Input: part model. Units: mm. Frame: model coordinates. A direction names the side the tool comes from. Coordinates: 2 decimals unless noted, no trailing zeros. Order: outer loops, then holes, each group sorted by start corner. A loop starts at its lowest first (then second) coordinate and runs counter-clockwise, first axis right, second up.
from build123d import *

# Parameters (mm, degrees)
SKETCH1_W           = 70
SKETCH1_H           = 30
BOSS_EXTRUDE1_DEPTH = 5
SKETCH2_W           = 70
SKETCH2_H           = 2
BOSS_EXTRUDE2_DEPTH = 50
SKETCH3_W           = 2
SKETCH3_H           = 26
BOSS_EXTRUDE3_DEPTH = 50
SKETCH4_W           = 42
SKETCH4_H           = 13
SKETCH4_W_2         = 40
SKETCH4_H_2         = 11
BOSS_EXTRUDE4_DEPTH = 40
SKETCH6_W           = 40
SKETCH6_H           = 40
CUT_EXTRUDE1_DEPTH  = 2
SKETCH7_W           = 15
SKETCH7_H           = 18
CUT_EXTRUDE2_DEPTH  = 5
SKETCH8_W           = 10
SKETCH8_H           = 10
CUT_EXTRUDE3_DEPTH  = 5


with BuildPart() as part:
    # Sketch1 → Boss-Extrude1 (new body)
    with BuildSketch(Plane(origin=(0, 0, 0), x_dir=(1, 0, 0), z_dir=(0, 1, 0))):
        Rectangle(SKETCH1_W, SKETCH1_H)
    extrude(amount=BOSS_EXTRUDE1_DEPTH)

    # Sketch2 → Boss-Extrude2 (add)
    with BuildSketch(Plane(origin=(0, 5, 0), x_dir=(1, 0, 0), z_dir=(0, 1, 0))):
        with Locations((0, -14)):
            Rectangle(SKETCH2_W, SKETCH2_H)
        with Locations((0, 14)):
            Rectangle(SKETCH2_W, SKETCH2_H)
    extrude(amount=BOSS_EXTRUDE2_DEPTH)

    # Sketch3 → Boss-Extrude3 (add)
    with BuildSketch(Plane(origin=(0, 5, 0), x_dir=(1, 0, 0), z_dir=(0, 1, 0))):
        with Locations((-34, 0)):
            Rectangle(SKETCH3_W, SKETCH3_H)
        with Locations((34, 0)):
            Rectangle(SKETCH3_W, SKETCH3_H)
    extrude(amount=BOSS_EXTRUDE3_DEPTH)

    # Sketch4 → Boss-Extrude4 (add)
    with BuildSketch(Plane(origin=(0, 5, 0), x_dir=(1, 0, 0), z_dir=(0, 1, 0))):
        Rectangle(SKETCH4_W, SKETCH4_H)
        Rectangle(SKETCH4_W_2, SKETCH4_H_2, mode=Mode.SUBTRACT)
    extrude(amount=BOSS_EXTRUDE4_DEPTH)

    # Sketch6 → Cut-Extrude1 (cut)
    with BuildSketch(Plane.XY.offset(6.5)):
        with Locations((0, 25)):
            Rectangle(SKETCH6_W, SKETCH6_H)
    extrude(amount=-CUT_EXTRUDE1_DEPTH, mode=Mode.SUBTRACT)

    # Sketch7 → Cut-Extrude2 (cut)
    with BuildSketch(Plane.XY.offset(15)):
        with Locations((-7.5, 36.5)):
            Rectangle(SKETCH7_W, SKETCH7_H)
        with Locations((7.5, 36.5)):
            Rectangle(SKETCH7_W, SKETCH7_H)
        with Locations((7.5, 18.5)):
            Rectangle(SKETCH7_W, SKETCH7_H)
        with Locations((-7.5, 18.5)):
            Rectangle(SKETCH7_W, SKETCH7_H)
    extrude(amount=-CUT_EXTRUDE2_DEPTH, mode=Mode.SUBTRACT)

    # Sketch8 → Cut-Extrude3 (cut)
    with BuildSketch(Plane.XZ):
        Rectangle(SKETCH8_W, SKETCH8_H)
    extrude(amount=-CUT_EXTRUDE3_DEPTH, mode=Mode.SUBTRACT)


solid = part.part
Item 1: Access query for faces 4 (the face through (0, 30, -13)), 5 (the face through (5, 2, 0)), 6 (the face through (15, 27, 14)). Directions: +Z, -Z, +X, -X, +Y, -Y. A direction counts if a zero-diameter tool reaches every point of the face in a straight line with its end or side. Return the directions, or none.
Response values:
face 4: +Y
face 5: +Y, -Y
face 6: +Z
Item 2: Cut plane D-D on x = 1. Return loops of the section in (y, z).
Response values:
outline: (0, -15) - (55, -15) - (55, -13) - (5, -13) - (5, -6.5) - (45, -6.5) - (45, -5.5) - (5, -5.5) - (5, -5) - (0, -5) - close; (0, 5) - (5, 5) - (5, 13) - (9.5, 13) - (9.5, 15) - (0, 15) - close; (45.5, 13) - (55, 13) - (55, 15) - (45.5, 15) - close
Item 3: Ray query, probe 1 along Z at (x, y) = (-19, 6.5); probe 2 along X at (y, z) = (42.5, 2.5); probe 3 along Z at (x, y) = (-2, 28). Return the intervals inside material, ascending.
Response values:
probe 1: z = -15 to -13, -6.5 to -5.5, 13 to 15
probe 2: x = -35 to -33, -21 to -20, 20 to 21, 33 to 35
probe 3: z = -15 to -13, -6.5 to -5.5
Item 4: Cut plane A-A on z = 0.5. Return loops of the section in (x, y).
Response values:
outline: (-35, 0) - (-5, 0) - (-5, 5) - (-20, 5) - (-20, 45) - (-21, 45) - (-21, 5) - (-33, 5) - (-33, 55) - (-35, 55) - close; (5, 0) - (35, 0) - (35, 55) - (33, 55) - (33, 5) - (21, 5) - (21, 45) - (20, 45) - (20, 5) - (5, 5) - close
Item 5: Cut plane B-B on y = 24.5. Return loops of the section in (x, z), then the cut area to 3 significant figures.
Response values:
outline: (-35, -15) - (35, -15) - (35, 15) - (15, 15) - (15, 13) - (33, 13) - (33, -13) - (-33, -13) - (-33, 13) - (-15, 13) - (-15, 15) - (-35, 15) - close; (-21, -6.5) - (21, -6.5) - (21, 6.5) - (20, 6.5) - (20, -5.5) - (-20, -5.5) - (-20, 6.5) - (-21, 6.5) - close
area: 390 mm2
Item 6: Cut plane C-C on x = 12. Return loops of the section in (y, z), then the cut area to 3 significant figures.
Response values:
outline: (0, -15) - (55, -15) - (55, -13) - (5, -13) - (5, -6.5) - (45, -6.5) - (45, -5.5) - (5, -5.5) - (5, 13) - (9.5, 13) - (9.5, 15) - (0, 15) - close; (45.5, 13) - (55, 13) - (55, 15) - (45.5, 15) - close
area: 318 mm2
Item 7: Draft query along Y for faces 1 (the face through (0, 0, -7)), 2 (the face through (0, 45.5, 14)), 3 (the face through (-33, 30, 0)). Return one class per face: pulls with the +Y half, pulls with the -Y half, needs draft (parallel to the pull), parting line crosses it, or undercut.
Response values:
face 1: pulls with the -Y half
face 2: undercut
face 3: needs draft
